Build history of the part. All positions in model axes, mm. A direction names the side the tool comes from. Give positions to 0.01 mm unless a question says otherwise; leave off trailing zeros. Order: outer loops, then holes, each group sorted by start corner. A loop starts at its lowest first (then second) coordinate and runs counter-clockwise, first axis right, second up. Notation, with made-up numbers: (46.25, 4) - (101.25, 4) arc R37 ccw to (101.25, 41) - close; hole circle Ø8 at (-21.75, 10.5). An arc over 180 degrees is marked (long way). Write each question's results on one line, items separated by ' | '. Start each with the question number.
Autodesk Fusion 360 part; units mm, degrees
sketch "Sketch1" plane through (0, 0, 0) normal (0, 0, 1) x (1, 0, 0)
  line L0 (-76.2, 0) -> (76.2, 0)
  line L1 (76.2, 0) -> (76.2, 57.15)
  line L2 (76.2, 57.15) -> (120.65, 57.15)
  line L3 (120.65, 57.15) -> (120.65, 127)
  line L4 (-0.5088, 127) -> (43.9412, 127)
  line L5 (43.9412, 127) -> (43.9412, 171.45)
  line L6 (43.9412, 171.45) -> (75.6912, 171.45)
  line L7 (75.6912, 171.45) -> (120.65, 127)
  line L8 (-0.5088, 127) -> (-44.9588, 127)
  line L9 (-44.9588, 127) -> (-44.9588, 171.45)
  line L10 (-44.9588, 171.45) -> (-76.7088, 171.45)
  line L11 (-76.2, 0) -> (-76.2, 57.15)
  line L12 (-76.2, 57.15) -> (-120.65, 57.15)
  line L13 (-120.65, 57.15) -> (-120.65, 127)
  line L14 (-120.65, 127) -> (-76.7088, 171.45)
  dimension "d1" = 57.15
  dimension "d2" = 44.45
  dimension "d3" = 69.85
  dimension "d4" = 44.45
  dimension "d5" = 44.45
  dimension "d6" = 31.75
  dimension "d7" = 44.45
  dimension "d8" = 44.45
  dimension "d9" = 31.75
  dimension "d10" = 57.15
  dimension "d11" = 44.45
  dimension "d12" = 69.85
extrude "Extrude1" add sketch "Sketch1" along normal blind 18.796
sketch "Sketch2" plane through (0, 0, 18.796) normal (0, 0, 1) x (1, 0, 0)
  line L0 (-76.2, 0) -> (76.2, 0)
  line L1 (76.2, 0) -> (76.2, 57.15)
  line L2 (76.2, 57.15) -> (120.65, 57.15)
  line L3 (120.65, 57.15) -> (120.65, 127)
  line L4 (120.65, 127) -> (75.6912, 171.45)
  line L5 (75.6912, 171.45) -> (43.9412, 171.45)
  line L6 (43.9412, 171.45) -> (43.9412, 127)
  line L7 (43.9412, 127) -> (-44.9588, 127)
  line L8 (-44.9588, 127) -> (-44.9588, 171.45)
  line L9 (-44.9588, 171.45) -> (-76.7088, 171.45)
  line L10 (-76.7088, 171.45) -> (-120.65, 127)
  line L11 (-120.65, 127) -> (-120.65, 57.15)
  line L12 (-120.65, 57.15) -> (-76.2, 57.15)
  line L13 (-76.2, 57.15) -> (-76.2, 0)
  circle A0 centre (-30.1503, 44.45) radius 4.7625
  circle A1 centre (29.7942, 44.45) radius 4.7625
  line L14 (0, 0) -> (-0.5088, 127)
  circle A2 centre (101.206, 98.552) radius 7.112
  circle A3 centre (-101.9956, 98.552) radius 7.112
  dimension "d15" = 9.525
  dimension "d16" = 9.525
  dimension "d17" = 44.45
  dimension "d18" = 29.972
  dimension "d19" = 29.972
  dimension "d20" = 44.45
  dimension "d21" = 14.224
  dimension "d22" = 14.224
  dimension "d23" = 101.6
  dimension "d24" = 98.552
  dimension "d25" = 101.6
  dimension "d26" = 98.552
sketch "Sketch3" plane through (76.2, 0, 0) normal (1, 0, 0) x (0, 0, -1)
  line L0 (0, 0) -> (0, 57.15)
  line L1 (0, 57.15) -> (-18.796, 57.15)
  line L2 (-18.796, 57.15) -> (-18.796, 0)
  line L3 (-18.796, 0) -> (0, 0)
  circle A0 centre (-9.3851, 44.45) radius 3.9624
  dimension "d27" = 7.9248
  dimension "d28" = 44.45
sketch "Sketch4" plane through (-76.2, 0, 0) normal (-1, 0, 0) x (0, 0, 1)
  line L0 (0, 57.15) -> (0, 0)
  line L1 (0, 0) -> (18.796, 0)
  line L2 (18.796, 0) -> (18.796, 57.15)
  line L3 (18.796, 57.15) -> (0, 57.15)
  circle A0 centre (9.3851, 44.45) radius 3.9624
sketch "Sketch5" plane through (0, 0, 0) normal (0, 0, -1) x (-1, 0, 0)
  line L0 (-76.2, 0) -> (76.2, 0)
  line L1 (76.2, 0) -> (76.2, 57.15)
  line L2 (76.2, 57.15) -> (120.65, 57.15)
  line L3 (120.65, 57.15) -> (120.65, 127)
  line L4 (120.65, 127) -> (76.7088, 171.45)
  line L5 (76.7088, 171.45) -> (44.9588, 171.45)
  line L6 (44.9588, 171.45) -> (44.9588, 127)
  line L7 (44.9588, 127) -> (-43.9412, 127)
  line L8 (-43.9412, 127) -> (-43.9412, 171.45)
  line L9 (-43.9412, 171.45) -> (-75.6912, 171.45)
  line L10 (-75.6912, 171.45) -> (-120.65, 127)
  line L11 (-120.65, 127) -> (-120.65, 57.15)
  line L12 (-120.65, 57.15) -> (-76.2, 57.15)
  line L13 (-76.2, 57.15) -> (-76.2, 0)
  circle A0 centre (-101.206, 98.552) radius 3.2004
  circle A1 centre (101.9956, 98.552) radius 3.2004
  dimension "d29" = 6.4008
  dimension "d30" = 6.4008
extrude "Extrude2" cut sketch "Sketch2" against normal blind 10.16 contours A0 | A1 | A2 | A3
extrude "Extrude3" cut 2 faces at (-29.7265, 42.4344, 8.636) (28.3639, 44.6971, 8.636) along direction (0, 0, -1) blind 48.26
extrude "Extrude4" cut sketch "Sketch5" against normal blind 8.636 contours A0 | A1
sketch "Sketch6" plane through (0, 0, 0) normal (0, -1, 0) x (1, 0, 0)
  line L0 (-76.2, 0) -> (76.2, 0)
  line L1 (76.2, 0) -> (76.2, 18.796)
  line L2 (76.2, 18.796) -> (-76.2, 18.796)
  line L3 (-76.2, 18.796) -> (-76.2, 0)
  circle A0 centre (0, 9.398) radius 3.9624
  circle A1 centre (44.45, 9.398) radius 3.9624
  circle A2 centre (-44.45, 9.398) radius 3.9624
  dimension "d37" = 7.9248
  dimension "d38" = 7.9248
  dimension "d39" = 7.9248
  dimension "d40" = 44.45
  dimension "d41" = 44.45
hole "Hole1" at (-44.45, 0, 9.398) at (0, 0, 9.398) at (44.45, 0, 9.398) direction (0, 1, 0) diameter 7.9248 depth 22.352 tip angle 118
hole "Hole2" at (76.2, 44.45, 9.3851) direction (-1, 0, 0) diameter 7.9248 depth 12.7 tip angle 118
hole "Hole3" at (-76.2, 44.45, 9.3851) direction (1, 0, 0) diameter 7.9248 depth 12.7 tip angle 118
sketch "Sketch7" plane through (0, 171.45, 0) normal (0, 1, 0) x (-1, 0, 0)
  line L0 (-75.6912, 0) -> (-43.9412, 0)
  line L1 (-43.9412, 0) -> (-43.9412, 18.796)
  line L2 (-43.9412, 18.796) -> (-75.6912, 18.796)
  line L3 (-75.6912, 18.796) -> (-75.6912, 0)
  circle A0 centre (-63.5, 9.3851) radius 3.175
  circle A1 centre (63.5, 9.3851) radius 3.175
  line L4 (63.5, 13.3475) -> (63.5, 5.4227)
  line L5 (76.2, 18.796) -> (-76.2, 18.796)
  line L6 (0, 0) -> (0, 18.796)
  dimension "d52" = 6.35
  dimension "d53" = 6.35
  dimension "d54" = 63.5
  dimension "d55" = 63.5
hole "Hole4" at (-63.5, 171.45, 9.3851) direction (0, -1, 0) diameter 6.35 depth 12.7 tip angle 118
sketch "Sketch8" plane through (0, 171.45, 0) normal (0, 1, 0) x (-1, 0, 0)
  line L0 (-75.6912, 0) -> (-43.9412, 0)
  line L1 (-43.9412, 0) -> (-43.9412, 18.796)
  line L2 (-43.9412, 18.796) -> (-75.6912, 18.796)
  line L3 (-75.6912, 18.796) -> (-75.6912, 0)
  circle A0 centre (-63.5, 8.6368) radius 3.175
  dimension "d59" = 6.35
  dimension "d60" = 127
hole "Hole5" at (63.5, 171.45, 8.6368) direction (0, -1, 0) diameter 6.35 depth 12.7 tip angle 118
thread "Thread1" thread offset 0 thread length 10.0076
thread "Thread2" thread offset 0 thread length 10.0076
thread "Thread3" thread offset 0 thread length 10.0076
thread "Thread4" thread offset 0 thread length 10.0076
thread "Thread5" thread offset 0 thread length 18.796
thread "Thread6" thread offset 0 thread length 18.796
Item 1: Cut at A-A, the plane x = -16.5. List the corners of the cut face in (y, z).
Item 2: Cut at B-B, the plane y = 37. List the corners of the cut face in (x, z).
Item 3: Two-plate mould, pull along Y, no slides. Class faces 4 (the cylindrical face through (96, 103.4, 13.8)), 5 (the flat face through (-44.959, 149, 9)), 6 (the cylindrical face through (-101.579, 101.725, 4.258)), 7 (the flat face through (-1, 0, 5)): +Y half, -Y half, draft (parallel to the pull), parting line (faces both ways), or undercut.
Item 4: Probe line 1 along Z through (x, y) = (0.5, 9); line 2 along Y through (x, z) = (-39, 15); line 3 along X through (y, z) = (154.5, 12.25). List the from-to ranges inside material, lowest first. Write a range as from..to.
Item 5: Which spindle directions (+Z, -Z, +X, -X, +Y, -Y) get a long thin tool onto all of the face, cutting with end or side? Do faces 1 (the flat face through (0, 127, 9)), 2 (the flat face through (98, 57.15, 9)), 3 (the flat face through (-98, 57.15, 9)). Say none if no direction does.
Item 6: Flat gauge pins, fed straight in: pin 1 Ø7 at (x, y) = (-100, 96.5) entering from +Z; pin 2 Ø1.5 at (x, y) = (66, 80.5) entering from -Z; pin 3 Ø6 at (y, z) = (19, 4.5) entering from +X; pin 4 Ø7 at (x, z) = (0, 9.398) entering from -Y. Where does each tip first touch, or does it go through?
Values found:
1) outline: (0, 0) - (127, 0) - (127, 18.8) - (0, 18.8) - close
2) outline: (-76.2, 0) - (76.2, 0) - (76.2, 18.8) - (-76.2, 18.8) - close
3) face 4: undercut | face 5: draft | face 6: undercut | face 7: -Y half
4) line 1: z = 0..5.47, 13.33..18.8 | line 2: y = 0..127 | line 3: x = -93.46..-44.96, 43.94..92.84
5) face 1: +Z, -Z, +Y | face 2: +Z, -Z, +X, -Y | face 3: +Z, -Z, -X, -Y
6) pin 1: stops at z = 8.64 | pin 2: stops at z = 0 | pin 3: stops at x = 76.2 | pin 4: stops at y = 22.63
